Read the model definition and answer for the solid it produces. Units are mm, in the model's axes. Coordinates: 2 decimals unless noted, no trailing zeros. Write each loop counter-clockwise with the first axis right and the second up, starting at its lowest first coordinate (ties: lowest second). Pieces come first, ordered by that corner, then holes.
1) The part is cut by section B-B (z = 4.2). Give the number of separate pieces and of enclosed holes in the cut face, then the cut area to 3 significant figures.
2) Each of these flat-tipped pins is pushed along its axis until it touches: pin 1 Ø1 at (y, z) = (6, 3) entering from -X; pin 2 Ø2 at (y, z) = (9, 2.5) entering from -X; pin 3 Ø1.5 at (x, z) = (131, 3) entering from +Y. Where does it stop, or does it pass through?
3) Find the intervals of material crossed by line 1 (X direction, y = -8, z = 1.1); line 2 (X direction, y = -6, z = 4); line 3 (Y direction, x = 154.5, z = 2.2), in increasing order.
4) The part is cut by section C-C (x = 52.5). Determine the outline of the cut face in (y, z) (3 decimals), then the cut area to 3 significant figures.
5) The part is cut by section A-A (x = 115). Determine the outline of the cut face in (y, z).
from build123d import *
from build123d.topology import SkipClean

# Parameters (mm, degrees)
EXTRUDE_3_DEPTH      = 5
SKETCH_4_R           = 4
SKETCH_4_R_2         = 1.5
CUT_EXTRUDE_3_DEPTH  = 5
SKETCH_5_R           = 11
CUT_EXTRUDE_4_DEPTH  = 2
SKETCH_6_R           = 1.5
CUT_EXTRUDE_6_DEPTH  = 169.745370307
SKETCH_7_R           = 1.5
CUT_EXTRUDE_7_DEPTH  = 10
SKETCH_8_R           = 11
CUT_EXTRUDE_8_DEPTH  = 10
SKETCH_9_R           = 1.5
CUT_EXTRUDE_9_DEPTH  = 10
SKETCH_10_R          = 5
CUT_EXTRUDE_10_DEPTH = 10
SKETCH_11_R          = 2
CUT_EXTRUDE_11_DEPTH = 10
SKETCH_12_W          = 41
SKETCH_12_H          = 22
CUT_EXTRUDE_12_DEPTH = 10


with BuildPart() as part:
    # 草图1 → 凸台-拉伸3 (new body)
    with BuildSketch(Plane.XY):
        with BuildLine():
            Line((140, 25), (0, 35))
            ThreePointArc((0, 35), (-35, 0), (0, -35))
            Line((0, -35), (140, -25))
            ThreePointArc((140, -25), (165, 0), (140, 25))
        make_face()
    extrude(amount=EXTRUDE_3_DEPTH)

    # 草图4 → 切除-拉伸3 (cut)
    with BuildSketch(Plane.XY.offset(5)):
        with Locations((140, 0)):
            Circle(SKETCH_4_R)
        Circle(SKETCH_4_R)
        with BuildLine():
            Line((-5, -3.5), (-5, -5))
            Line((-5, -5), (-3.5, -5))
            ThreePointArc((-3.5, -5), (-3.939339828, -3.939339828), (-5, -3.5))
        make_face()
        with BuildLine():
            Line((-3.5, -5), (-5, -5))
            Line((-5, -5), (-5, -3.5))
            ThreePointArc((-5, -3.5), (-6.060660172, -6.060660172), (-3.5, -5))
        make_face()
        with Locations((135, 5)):
            Circle(SKETCH_4_R_2)
        with Locations((135, -5)):
            Circle(SKETCH_4_R_2)
        with Locations((145, -5)):
            Circle(SKETCH_4_R_2)
        with Locations((145, 5)):
            Circle(SKETCH_4_R_2)
        with Locations((-5, 5)):
            Circle(SKETCH_4_R_2)
        with Locations((5, 5)):
            Circle(SKETCH_4_R_2)
        with Locations((5, -5)):
            Circle(SKETCH_4_R_2)
    extrude(amount=-CUT_EXTRUDE_3_DEPTH, mode=Mode.SUBTRACT)

    # 草图5 → 切除-拉伸4 (cut)
    with BuildSketch(Plane.XY.offset(5)):
        Circle(SKETCH_5_R)
        with Locations((140, 0)):
            Circle(SKETCH_5_R)
    extrude(amount=-CUT_EXTRUDE_4_DEPTH, mode=Mode.SUBTRACT)

    # 草图6 → 切除-拉伸6 (cut, through all)
    with BuildSketch(Plane.XY.offset(5)):
        with Locations((0, 30)):
            Circle(SKETCH_6_R)
        with Locations((15, 25.980762114)):
            Circle(SKETCH_6_R)
        with Locations((25.980762114, 15)):
            Circle(SKETCH_6_R)
        with Locations((30, 0)):
            Circle(SKETCH_6_R)
        with Locations((25.980762114, -15)):
            Circle(SKETCH_6_R)
        with Locations((15, -25.980762114)):
            Circle(SKETCH_6_R)
        with Locations((0, -30)):
            Circle(SKETCH_6_R)
        with Locations((-15, -25.980762114)):
            Circle(SKETCH_6_R)
        with Locations((-25.980762114, -15)):
            Circle(SKETCH_6_R)
        with Locations((-30, 0)):
            Circle(SKETCH_6_R)
        with Locations((-25.980762114, 15)):
            Circle(SKETCH_6_R)
        with Locations((-15, 25.980762114)):
            Circle(SKETCH_6_R)
        with Locations((140, 20)):
            Circle(SKETCH_6_R)
        with Locations((150, 17.320508076)):
            Circle(SKETCH_6_R)
        with Locations((157.320508076, 10)):
            Circle(SKETCH_6_R)
        with Locations((160, 0)):
            Circle(SKETCH_6_R)
        with Locations((157.320508076, -10)):
            Circle(SKETCH_6_R)
        with Locations((150, -17.320508076)):
            Circle(SKETCH_6_R)
        with Locations((140, -20)):
            Circle(SKETCH_6_R)
        with Locations((130, -17.320508076)):
            Circle(SKETCH_6_R)
        with Locations((122.679491924, -10)):
            Circle(SKETCH_6_R)
        with Locations((120, 0)):
            Circle(SKETCH_6_R)
        with Locations((122.679491924, 10)):
            Circle(SKETCH_6_R)
        with Locations((130, 17.320508076)):
            Circle(SKETCH_6_R)
    extrude(amount=-CUT_EXTRUDE_6_DEPTH, mode=Mode.SUBTRACT)

    # 草图7 → 切除-拉伸7 (cut)
    with SkipClean():  # the faces are left unmerged after this step: merging them gives an invalid solid
        with BuildSketch(Plane.XY.offset(5)):
            with BuildLine():
                ThreePointArc((138.21656051, 24.936305732), (139.107711737, 24.984071359), (140, 25))
                Line((140, 25), (0, 35))
                ThreePointArc((0, 35), (-35, 0), (0, -35))
                Line((0, -35), (140, -25))
                ThreePointArc((140, -25), (139.107711737, -24.984071359), (138.21656051, -24.936305732))
                Line((138.21656051, -24.936305732), (0, -20))
                ThreePointArc((0, -20), (-20, 0), (0, 20))
                Line((0, 20), (138.21656051, 24.936305732))
            make_face()
            with Locations((0, -30)):
                Circle(SKETCH_7_R, mode=Mode.SUBTRACT)
            with Locations((-15, -25.980762114)):
                Circle(SKETCH_7_R, mode=Mode.SUBTRACT)
            with Locations((15, -25.980762114)):
                Circle(SKETCH_7_R, mode=Mode.SUBTRACT)
            with Locations((-25.980762114, -15)):
                Circle(SKETCH_7_R, mode=Mode.SUBTRACT)
            with Locations((-30, 0)):
                Circle(SKETCH_7_R, mode=Mode.SUBTRACT)
            with Locations((-25.980762114, 15)):
                Circle(SKETCH_7_R, mode=Mode.SUBTRACT)
            with Locations((-15, 25.980762114)):
                Circle(SKETCH_7_R, mode=Mode.SUBTRACT)
            with Locations((0, 30)):
                Circle(SKETCH_7_R, mode=Mode.SUBTRACT)
            with Locations((15, 25.980762114)):
                Circle(SKETCH_7_R, mode=Mode.SUBTRACT)
        extrude(amount=-CUT_EXTRUDE_7_DEPTH, mode=Mode.SUBTRACT)

    # 草图8 → 切除-拉伸8 (cut)
    with SkipClean():  # the faces are left unmerged after this step: merging them gives an invalid solid
        with BuildSketch(Plane.XY.offset(5)):
            Circle(SKETCH_8_R)
        extrude(amount=-CUT_EXTRUDE_8_DEPTH, mode=Mode.SUBTRACT)

    # 草图9 → 切除-拉伸9 (cut)
    with SkipClean():  # the faces are left unmerged after this step: merging them gives an invalid solid
        with BuildSketch(Plane.XY.offset(5)):
            with Locations((0, 15)):
                Circle(SKETCH_9_R)
            with Locations((10.606601718, 10.606601718)):
                Circle(SKETCH_9_R)
            with Locations((15, 0)):
                Circle(SKETCH_9_R)
            with Locations((10.606601718, -10.606601718)):
                Circle(SKETCH_9_R)
            with Locations((0, -15)):
                Circle(SKETCH_9_R)
            with Locations((-10.606601718, -10.606601718)):
                Circle(SKETCH_9_R)
            with Locations((-15, 0)):
                Circle(SKETCH_9_R)
            with Locations((-10.606601718, 10.606601718)):
                Circle(SKETCH_9_R)
        extrude(amount=-CUT_EXTRUDE_9_DEPTH, mode=Mode.SUBTRACT)

    # 草图10 → 切除-拉伸10 (cut)
    with SkipClean():  # the faces are left unmerged after this step: merging them gives an invalid solid
        with BuildSketch(Plane.XY.offset(3)):
            with Locations((140, 0)):
                Circle(SKETCH_10_R)
        extrude(amount=-CUT_EXTRUDE_10_DEPTH, mode=Mode.SUBTRACT)

    # 草图11 → 切除-拉伸11 (cut)
    with SkipClean():  # the faces are left unmerged after this step: merging them gives an invalid solid
        with BuildSketch(Plane.XY.offset(5)):
            with Locations((105.5, 5)):
                Circle(SKETCH_11_R)
            Polygon((110, 10), (110, 0), (110, -10), (150, -10), (150, 10), align=None)
            with Locations((105.5, -5)):
                Circle(SKETCH_11_R)
            with Locations((154.5, -5)):
                Circle(SKETCH_11_R)
            with Locations((154.5, 5)):
                Circle(SKETCH_11_R)
        extrude(amount=-CUT_EXTRUDE_11_DEPTH, mode=Mode.SUBTRACT)

    # 草图12 → 切除-拉伸12 (cut)
    with SkipClean():  # the faces are left unmerged after this step: merging them gives an invalid solid
        with BuildSketch(Plane.XY.offset(5)):
            with Locations((130, 0)):
                Rectangle(SKETCH_12_W, SKETCH_12_H)
        extrude(amount=-CUT_EXTRUDE_12_DEPTH, mode=Mode.SUBTRACT)


solid = part.part
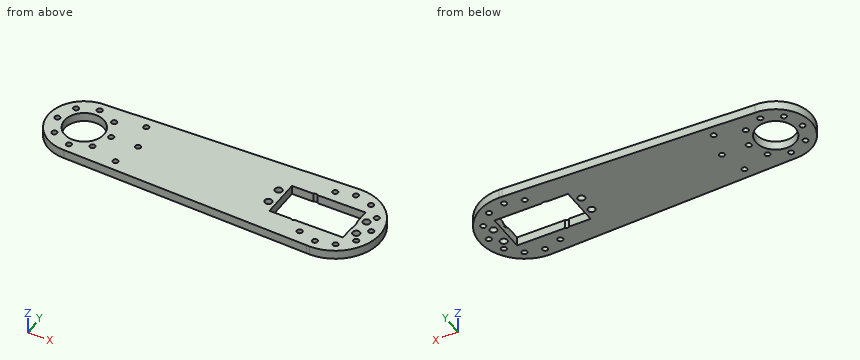
Reported:
1. separate pieces: 1
1. enclosed holes: 26
1. area: 6,430 mm2
2. pin 1: stops at x = -19.23
2. pin 2: stops at x = -18.33
2. pin 3: stops at y = 24.71
3. line 1: x = -18.33 to -7.55, 7.55 to 109.5, 150.5 to 163.69
3. line 2: x = -19.08 to -9.22, 9.22 to 103.77, 107.23 to 109.5, 150.5 to 152.77, 156.23 to 164.27
3. line 3: y = -20.37 to -7, -3 to 3, 7 to 20.37
4. outline: (-21.875, 0) - (21.875, 0) - (21.875, 5) - (-21.875, 5) - close
4. area: 219 mm2
5. outline: (-24.11, 0) - (-11, 0) - (-11, 5) - (-24.11, 5) - close; (11, 0) - (24.11, 0) - (24.11, 5) - (11, 5) - close
